Design review of the part built by this model. Coordinates are the model's own, in mm. A direction names the side the tool comes from. Round coordinates to 2 decimals unless told otherwise and drop trailing zeros. Loops run counter-clockwise (first coordinate to the right, second up) from the corner with the lowest first, then second, coordinate; pieces in that order, holes last. Notation, with made-up numbers: (-17, 85) - (1, 85) arc R20 cw to (1, 94) - close; hole circle Ø10 at (-8.5, 57.25). An arc over 180 degrees is marked (long way). Return JSON: item names as keys, results as strings. Group by question number.
(1) Clearance check with flat-ended pins moving along their axes: pin 1 (6 mm diameter, centred on y = 7, z = 95, fed in from -X); pin 2 (1.5 mm diameter, centred on y = 214, z = 361.5, fed in from +X); pin 3 (10 mm diameter, centred on y = -854, z = 228, fed in from -X). State where each tip first meets the part, or that it passes through.
(2) Wall thickness on L1, parallel to Y at x = 41.5, z = 392.5; L2, parallel to Y at x = 684, z = 107; L3, parallel to X at y = -615, z = 121: over which ranges is each line inside the solid? List them lowest first. Write a range as [from, to].
(3) For faces 4 (the flat face through (-95.99, 740.33, 135.39)), 5 (the cylindrical face through (316.16, -587.26, 156.88)), 6 (the flat face through (-103.197, 1339.435, 246.5)), list the 3-axis set-ups (+Z, -Z, +X, -X, +Y, -Y) from which the entire face can be reached by the end or side of a thin tool; tool diameter is ignored.
(4) We need section A-A, the plane z = 60. Write out the cut boundary in (x, y), and give its area (3 significant figures).
(5) The part is to be moulded in two halves that separate along Y. For faces 1 (the cylindrical face through (-46.54, 459.03, 156.92)), 2 (the flat face through (114, -120, 0)), 3 (the flat face through (-77.624, 1504.86, 246.5)), say which applies: pulls with the +Y half, pulls with the -Y half, needs draft (parallel to the pull), parting line crosses it, or undercut.
from build123d import *

# Parameters (mm, degrees)
F1_DEPTH = 500
F2_R     = 48.0212425181
F2_R_2   = 56.0010929185
F2_R_3   = 109.5030020502
F2_R_4   = 58.0607354524
F2_R_5   = 53.7611851769
F3_DEPTH = 50
F5_DEPTH = 500
F6_R     = 60.7396670844
F6_R_2   = 74.2371640954
F6_R_3   = 52.0726222856
F6_R_4   = 59.6000564376
F6_R_5   = 119.2001237969
F7_DEPTH = 100


# Not quite as in the source:
# - a feature names something its author has since deleted; it is built from what else it names


with BuildPart() as f1:
    # F0 (on Top) → F1 (new body)
    with BuildSketch(Plane.XY):
        with BuildLine():
            ThreePointArc((-16.3297786736, 125.9457753498), (-2.847496792, 126.9680737903), (10.6670605483, 126.5512300187))
            Line((10.6670605483, 126.5512300187), (-137.3067498207, 1246.1612224579))
            Line((-137.3067498207, 1246.1612224579), (-68.1192024335, 1435.3577301921))
            Line((-68.1192024335, 1435.3577301921), (-87.3996093869, 1576.3362646103))
            Line((-87.3996093869, 1576.3362646103), (-173.4057664871, 1337.4170064926))
            Line((-173.4057664871, 1337.4170064926), (-16.3297786736, 125.9457753498))
        make_face()
        with BuildLine():
            ThreePointArc((-16.3297786736, 125.9457753498), (-83.8305377188, -95.4014724508), (127, 0))
            ThreePointArc((127, 0), (93.4979055638, 85.9484825647), (10.6670605483, 126.5512300187))
            ThreePointArc((10.6670605483, 126.5512300187), (-2.847496792, 126.9680737903), (-16.3297786736, 125.9457753498))
        make_face()
    extrude(amount=F1_DEPTH)

    # F2 (on face) → F3 (cut)
    with BuildSketch(Plane(origin=(0, 0, 0), x_dir=(0.1285809344, -0.9916990185, 0), z_dir=(-0.9916990185, -0.1285809344, 0))):
        with Locations((-1136.4312171936, 425.6200194359)):
            Circle(F2_R)
        with Locations((-933.0058097839, 387.370377779)):
            Circle(F2_R_2)
        with Locations((-711.0854387283, 287.7508103848)):
            Circle(F2_R_3)
        with Locations((-487.9950881004, 208.4301263094)):
            Circle(F2_R_4)
        with Locations((-284.7935259342, 177.8837442398)):
            Circle(F2_R_5)
    extrude(amount=-F3_DEPTH, mode=Mode.SUBTRACT)

    # F4 (on face) → F5 (join)
    with BuildSketch(Plane(origin=(0, 0, 0), x_dir=(1, 0, 0), z_dir=(0, 0, -1))):
        with BuildLine():
            Line((517.1427625415, 1082.8496493747), (54.8823102258, 114.918538341))
            ThreePointArc((54.8823102258, 114.918538341), (83.4911676886, 96.1642519242), (106.0759476154, 70.4714961361))
            Line((106.0759476154, 70.4714961361), (560.7657432556, 1022.5503444672))
            Line((560.7657432556, 1022.5503444672), (699.5562911034, 1082.8496493747))
            Line((699.5562911034, 1082.8496493747), (744.8581457138, 1188.7502670288))
            Line((744.8581457138, 1188.7502670288), (517.1427625415, 1082.8496493747))
        make_face()
        with BuildLine():
            ThreePointArc((106.0759476154, 70.4714961361), (83.4911676886, 96.1642519242), (54.8823102258, 114.918538341))
            ThreePointArc((54.8823102258, 114.918538341), (-107.7210952255, -67.9301411273), (127.3512403951, 0))
            ThreePointArc((127.3512403951, 0), (121.9164507666, 36.8064866923), (106.0759476154, 70.4714961361))
        make_face()
    extrude(amount=-F5_DEPTH)

    # F6 (on face) → F7 (cut)
    with BuildSketch(Plane(origin=(0, 0, 0), x_dir=(0.4309523021, -0.9023747078, 0), z_dir=(-0.9023747078, -0.4309523021, 0))):
        with Locations((282.9372286797, 154.2636454105)):
            Circle(F6_R)
        with Locations((903.6465287209, 359.3041300774)):
            Circle(F6_R_2)
        with Locations((1114.4098043442, 373.2200860977)):
            Circle(F6_R_3)
        with Locations((504.1354894638, 163.9334559441)):
            Circle(F6_R_4)
        with Locations((692.0155882835, 273.2473611832)):
            Circle(F6_R_5)
    extrude(amount=-F7_DEPTH, mode=Mode.SUBTRACT)


solid = f1.part
Solutions:
{
 "1": {"pin 1": "x = -127.29", "pin 2": "x = -0.79", "pin 3": "x = 405.46"},
 "2": {"L1": "[-120.4, 120.4]", "L2": "[-1160.45, -1076.09]", "L3": "[293.71, 366.13]"},
 "3": {"face 4": "+Z, -Z, -X", "face 5": "none", "face 6": "+Z, -Z, +X"},
 "4": {"outline": "(-173.41, 1337.42) - (-16.37, 126.29) arc R127.35 ccw (long way) to (54.88, -114.92) - (517.14, -1082.85) - (744.86, -1188.75) - (699.56, -1082.85) - (560.77, -1022.55) - (106.08, -70.47) arc R127.35 ccw to (10.62, 126.91) - (-137.31, 1246.16) - (-68.12, 1435.36) - (-87.4, 1576.34) - close", "area": "180,000 mm^2"},
 "5": {"face 1": "undercut", "face 2": "needs draft", "face 3": "pulls with the +Y half"}
}
